Input: part model. Units: mm. Frame: model coordinates. Round coordinates to 2 decimals unless told otherwise and drop trailing zeros. Loops run counter-clockwise (first coordinate to the right, second up) from the corner with the lowest first, then second, coordinate; pieces in that order, holes last. Notation, with made-up numbers: (8, 53) - (20, 53) arc R26 ccw to (20, 72) - close; hole circle Ø3 at (72.5, -28). An arc over 180 degrees is marked (long way). Use CSV: the item, a comma, the result in double quotes. Start each with the question number.
1. Cut plane C-C (z = 0.5). Give the number of separate pieces and of enclosed holes in the cut face, and give its area (3 significant figures).
2. Cut plane B-B (x = 23.25). Return loops of the section in (y, z), and give its area (3 significant figures).
3. Pin query (flat end, axial travel): P1, Ø1.5, axis at y = -16, z = 1.5, coming from the +X side; P2, Ø1.5, axis at y = 1.5, z = 1, coming from the -X side; P3, Ø0.9, axis at x = -47, z = 1.5, coming from the -Y side; P4, Ø7, axis at x = -69.75, y = 10, coming from the -Z side. Return the tip coordinate at first contact, or that it passes through.
4. Material intervals for probe 1 along Y at (x, z) = (-69.75, 1.2); probe 2 along X at (y, z) = (1, 1.95); probe 3 along X at (y, z) = (13, 2.5), sorted ascending. Write a range as from..to.
5. Cut plane A-A (y = -5). Return loops of the section in (x, z).
6. Cut plane D-D (y = -16.5). Return loops of the section in (x, z), and give its area (3 significant figures).
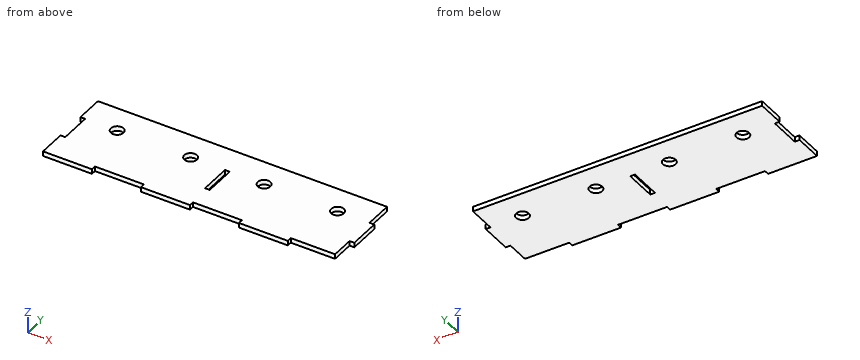
```python
from build123d import *

# Parameters (mm, degrees)
SKETCH1_R           = 4
SKETCH1_W           = 3
SKETCH1_H           = 20
BOSS_EXTRUDE1_DEPTH = 3


with BuildPart() as part:
    # Sketch1 → Boss-Extrude1 (new body)
    with BuildSketch(Plane.XY):
        Polygon((-93, 27.5), (-93, 10), (-90, 10), (-90, -10), (-93, -10), (-93, -27.5), (-62, -27.5), (-62, -24.5), (-31, -24.5), (-31, -27.5), (0, -27.5), (0, -24.5), (31, -24.5), (31, -27.5), (62, -27.5), (62, -24.5), (90, -24.5), (90, -10), (93, -10), (93, 10), (90, 10), (90, 27.5), (0, 27.5), align=None)
        with Locations((-69.75, 10)):
            Circle(SKETCH1_R, mode=Mode.SUBTRACT)
        Rectangle(SKETCH1_W, SKETCH1_H, mode=Mode.SUBTRACT)
        with Locations((-23.25, 10)):
            Circle(SKETCH1_R, mode=Mode.SUBTRACT)
        with Locations((23.25, 10)):
            Circle(SKETCH1_R, mode=Mode.SUBTRACT)
        with Locations((69.75, 10)):
            Circle(SKETCH1_R, mode=Mode.SUBTRACT)
    extrude(amount=BOSS_EXTRUDE1_DEPTH)


solid = part.part
```
Established:
1,separate pieces,"1"
1,enclosed holes,"5"
1,area,"9,530 mm2"
2,outline,"(-24.5, 0) - (6, 0) - (6, 3) - (-24.5, 3) - close; (14, 0) - (27.5, 0) - (27.5, 3) - (14, 3) - close"
2,area,"132 mm2"
3,P1,"stops at x = 90"
3,P2,"stops at x = -90"
3,P3,"stops at y = -24.5"
3,P4,"passes through"
4,probe 1,"y = -27.5..6, 14..27.5"
4,probe 2,"x = -90..-1.5, 1.5..93"
4,probe 3,"x = -93..-72.4, -67.1..-25.9, -20.6..20.6, 25.9..67.1, 72.4..90"
5,outline,"(-90, 0) - (-1.5, 0) - (-1.5, 3) - (-90, 3) - close; (1.5, 0) - (93, 0) - (93, 3) - (1.5, 3) - close"
6,outline,"(-93, 0) - (90, 0) - (90, 3) - (-93, 3) - close"
6,area,"549 mm2"
